Source: CAD feature listing. Evaluate the final solid. Frame: model axes, mm. A direction names the side the tool comes from. Round coordinates to 2 decimals unless told otherwise and drop trailing zeros. Order: outer loops, then holes, each group sorted by start corner. A loop starts at its lowest first (then second) coordinate and runs counter-clockwise, first axis right, second up. Notation, with made-up numbers: M 38.25,77 L 83.25,77 A9 cw 83.25,88 Z; hole C -17,-25 d10. An arc over 180 degrees is marked long. Answer as CSV lines item,"result". Start each with the question number.
Item 1: Section query A-A on x = -25. State how many separate pieces and enclosed holes the cut face has, plus the area to 3 significant figures.
Item 2: Section query B-B on x = -14.5. Return the cut outline in (y, z), plus the area to 3 significant figures.
Item 3: First-contact query: P1, Ø8, axis at x = -17, z = 9, coming from the +Y side; P2, Ø0.8, axis at x = 37, y = -19.5, coming from the +Z side; P3, Ø2.5, axis at x = 25, y = 29.5, coming from the +Z side; P4, Ø13, axis at x = 8.5, z = 8.5, coming from the -Y side. Flat tips, straight axial feed; report the tip coordinate or a pass-through.
Item 4: Pull-direction query (X, two-part tool) for faces 6 (the face through (36.86, -0.9, 18.11)), 7 (the face through (-34.577, 23.748, -1.787)), 8 (the face through (44.748, 11.112, -1.787)); classes: +X half, -X half, draft (parallel to the pull), parting line (faces both ways), or undercut.
Item 5: Section query C-C on x = -2. Return the cut outline in (y, z), plus the area to 3 significant figures.
Item 6: Line query: line 1 (Y direction, x = -33.5, z = 18.25); line 2 (Y direction, x = 25, z = -1.5); line 3 (X direction, y = 3.5, z = 24.75). Output: solid intervals per line, ascending. Write a range as [from, to].
Item 7: Set-up query: faces 1 (the face through (40.96, 18.61, 11.34)), 2 (the face through (43.93, 22.85, 13.18)), 3 (the face through (-24, 27, 0)), 4 (the face through (-26.11, 28.49, -1.76)), 5 (the face through (38.5, -21, 10)). Return all of +Z, -Z, +X, -X, +Y, -Y with unobstructed straight access to the full face (end or side cutting, diameter ignored); none if empty.
from build123d import *

# Parameters (mm, degrees)
PAD_DEPTH       = 26
FILLET_R        = 3
THICKNESS_T     = 2.5
SKETCH001_R     = 2.5
SKETCH001_R_2   = 1
PAD001_DEPTH    = 4
SKETCH007_W     = 19
SKETCH007_H     = 8
POCKET_DEPTH    = 5
PAD008_DEPTH    = 10
SKETCH013_W     = 22
SKETCH013_H     = 10
POCKET002_DEPTH = 5
SKETCH014_W     = 24
SKETCH014_H     = 10
POCKET003_DEPTH = 5
FILLET001_R     = 2
FILLET002_R     = 2
FILLET003_R     = 2
SKETCH015_W     = 5
SKETCH015_H     = 5
SKETCH015_R     = 1
PAD011_DEPTH    = 24
SKETCH016_R     = 1.5
PAD012_DEPTH    = 2.5
CHAMFER_SIZE    = 1
CHAMFER001_SIZE = 1
CHAMFER002_SIZE = 1


with BuildPart() as part:
    # Sketch → Pad (new body)
    with BuildSketch(Plane.XY):
        Polygon((-43, 22), (-43, 0), (-36, 0), (-36, -41), (36, -41), (36, 0), (43, 0), (43, 22), align=None)
    extrude(amount=PAD_DEPTH)

    # Fillet
    fillet_edges = [part.edges().sort_by_distance(p)[0] for p in [
        (-36, -41, 13),
        (36, -41, 13),
        (43, 0, 13),
        (-43, 0, 13),
        (-43, 22, 13),
        (43, 22, 13),
        (36, 0, 13),
        (-36, 0, 13),
    ]]
    fillet(fillet_edges, radius=FILLET_R)

    # Thickness
    thickness_openings = [part.faces().sort_by_distance(p)[0] for p in [
        (0, -8.19552, 26),
    ]]
    offset(amount=THICKNESS_T, openings=thickness_openings)

    # Sketch001 (on Face2 of Thickness) → Pad001 (join)
    with BuildSketch(Plane.XY):
        with Locations((-32.7, -6.5)):
            Circle(SKETCH001_R)
        with Locations((-32.7, -6.5)):
            Circle(SKETCH001_R_2, mode=Mode.SUBTRACT)
        with Locations((-32.7, -32.7)):
            Circle(SKETCH001_R)
        with Locations((-32.7, -32.7)):
            Circle(SKETCH001_R_2, mode=Mode.SUBTRACT)
        with Locations((32.7, -32.7)):
            Circle(SKETCH001_R)
        with Locations((32.7, -32.7)):
            Circle(SKETCH001_R_2, mode=Mode.SUBTRACT)
        with Locations((32.7, -6.5)):
            Circle(SKETCH001_R)
        with Locations((32.7, -6.5)):
            Circle(SKETCH001_R_2, mode=Mode.SUBTRACT)
    extrude(amount=PAD001_DEPTH)

    # Sketch007 (on Face24 of Pad001) → Pocket (cut)
    with BuildSketch(Plane.YZ.offset(38.5)):
        with Locations((-20.85, 22)):
            Rectangle(SKETCH007_W, SKETCH007_H)
    extrude(amount=-POCKET_DEPTH, mode=Mode.SUBTRACT)

    # Sketch009 (on Face2 of Pocket) → Pad008 (join)
    with BuildSketch(Plane.XY):
        Polygon((43, 5), (37.6, 5), (37.6, 1), (30.6, 1), (30.6, -3), (37.6, -3), (43, 0), align=None)
        Polygon((-43, 5), (-37.6, 5), (-37.6, 1), (-30.6, 1), (-30.6, -3), (-37.6, -3), (-43, 0), align=None)
    extrude(amount=PAD008_DEPTH)

    # Sketch013 → Pocket002 (cut)
    with BuildSketch(Plane.XZ.offset(43.5)):
        with Locations((-19, 14.5)):
            Rectangle(SKETCH013_W, SKETCH013_H)
    extrude(amount=-POCKET002_DEPTH, mode=Mode.SUBTRACT)

    # Sketch014 (on Face36 of Pocket002) → Pocket003 (cut)
    with BuildSketch(Plane(origin=(-38.5, 0, 0), x_dir=(0, -1, 0), z_dir=(-1, 0, 0))):
        with Locations((15, 8.5)):
            Rectangle(SKETCH014_W, SKETCH014_H)
    extrude(amount=-POCKET003_DEPTH, mode=Mode.SUBTRACT)

    # Fillet001
    fillet001_edges = [part.edges().sort_by_distance(p)[0] for p in [
        (-37.25, -3, 13.5),
        (-37.25, -3, 3.5),
        (-37.25, -27, 13.5),
        (-37.25, -27, 3.5),
    ]]
    fillet(fillet001_edges, radius=FILLET001_R)

    # Fillet002
    fillet002_edges = [part.edges().sort_by_distance(p)[0] for p in [
        (-30, -42.25, 9.5),
        (-30, -42.25, 19.5),
        (-8, -42.25, 19.5),
        (-8, -42.25, 9.5),
    ]]
    fillet(fillet002_edges, radius=FILLET002_R)

    # Fillet003
    fillet003_edges = [part.edges().sort_by_distance(p)[0] for p in [
        (37.25, -30.35, 18),
        (37.25, -11.35, 18),
    ]]
    fillet(fillet003_edges, radius=FILLET003_R)

    # Sketch015 (on Face10 of Fillet003) → Pad011 (join)
    with BuildSketch(Plane.XY):
        with Locations((-40.5, 19.5)):
            Rectangle(SKETCH015_W, SKETCH015_H)
        with Locations((-40.5, 19.5)):
            Circle(SKETCH015_R, mode=Mode.SUBTRACT)
        with Locations((40.5, 19.5)):
            Rectangle(SKETCH015_W, SKETCH015_H)
        with Locations((40.5, 19.5)):
            Circle(SKETCH015_R, mode=Mode.SUBTRACT)
        with Locations((33.5, -38.5)):
            Rectangle(SKETCH015_W, SKETCH015_H)
        with Locations((33.5, -38.5)):
            Circle(SKETCH015_R, mode=Mode.SUBTRACT)
        with Locations((-33.5, -38.5)):
            Rectangle(SKETCH015_W, SKETCH015_H)
        with Locations((-33.5, -38.5)):
            Circle(SKETCH015_R, mode=Mode.SUBTRACT)
    extrude(amount=PAD011_DEPTH)

    # Sketch016 (on Face110 of Pad011) → Pad012 (join)
    with BuildSketch(Plane(origin=(0, 0, -2.5), x_dir=(1, 0, 0), z_dir=(0, 0, -1))):
        with BuildLine():
            ThreePointArc((-20, 48.5), (-25, 53.5), (-30, 48.5))
            Line((-30, 48.5), (-30, 38.5))
            ThreePointArc((-30, 38.5), (-25, 33.5), (-20, 38.5))
            Line((-20, 48.5), (-20, 38.5))
        make_face()
        with Locations((-25, 48.5)):
            Circle(SKETCH016_R, mode=Mode.SUBTRACT)
        with BuildLine():
            ThreePointArc((30, 48.5), (25, 53.5), (20, 48.5))
            Line((20, 48.5), (20, 38.5))
            ThreePointArc((20, 38.5), (25, 33.5), (30, 38.5))
            Line((30, 48.5), (30, 38.5))
        make_face()
        with Locations((25, 48.5)):
            Circle(SKETCH016_R, mode=Mode.SUBTRACT)
        with BuildLine():
            ThreePointArc((-20, -19.5), (-25, -14.5), (-30, -19.5))
            Line((-30, -19.5), (-30, -29.5))
            ThreePointArc((-30, -29.5), (-25, -34.5), (-20, -29.5))
            Line((-20, -19.5), (-20, -29.5))
        make_face()
        with Locations((-25, -29.5)):
            Circle(SKETCH016_R, mode=Mode.SUBTRACT)
        with BuildLine():
            ThreePointArc((30, -19.5), (25, -14.5), (20, -19.5))
            Line((20, -19.5), (20, -29.5))
            ThreePointArc((20, -29.5), (25, -34.5), (30, -29.5))
            Line((30, -19.5), (30, -29.5))
        make_face()
        with Locations((25, -29.5)):
            Circle(SKETCH016_R, mode=Mode.SUBTRACT)
    extrude(amount=-PAD012_DEPTH)

    # Chamfer
    chamfer_edges = [part.edges().sort_by_distance(p)[0] for p in [
        (-20, -46, 0),
        (20, -46, 0),
        (-30, 27, 0),
        (20, 27, 0),
        (23.5, 29.5, 0),
        (-26.5, 29.5, 0),
        (-26.5, -48.5, 0),
        (23.5, -48.5, 0),
    ]]
    chamfer(chamfer_edges, length=CHAMFER_SIZE)

    # Chamfer001
    chamfer001_edges = [part.edges().sort_by_distance(p)[0] for p in [
        (-41.5, 19.5, 24),
        (39.5, 19.5, 24),
        (32.5, -38.5, 24),
        (-34.5, -38.5, 24),
    ]]
    chamfer(chamfer001_edges, length=CHAMFER001_SIZE)

    # Chamfer002
    chamfer002_edges = [part.edges().sort_by_distance(p)[0] for p in [
        (-37.6, 3, 10),
        (-34.1, 1, 10),
        (34.1, 1, 10),
        (37.6, 3, 10),
    ]]
    chamfer(chamfer002_edges, length=CHAMFER002_SIZE)


solid = part.part
Results:
1,separate pieces,"4"
1,enclosed holes,"0"
1,area,"307 mm^2"
2,outline,"M -43.5,0 A2.5 ccw -41,-2.5 L 22,-2.5 A2.5 ccw 24.5,0 L 24.5,26 L 22,26 L 22,0 L -41,0 L -41,9.5 L -43.5,9.5 Z; M -43.5,19.5 L -41,19.5 L -41,26 L -43.5,26 Z"
2,area,"272 mm^2"
3,P1,"y = 24.5"
3,P2,"z = 18"
3,P3,"through"
3,P4,"y = -43.5"
4,face 6,"undercut"
4,face 7,"draft"
4,face 8,"+X half"
5,outline,"M -43.5,0 A2.5 ccw -41,-2.5 L 22,-2.5 A2.5 ccw 24.5,0 L 24.5,26 L 22,26 L 22,0 L -41,0 L -41,26 L -43.5,26 Z"
5,area,"297 mm^2"
6,line 1,"[-43.48, -39.5], [-37.5, -36], [22, 24.5]"
6,line 2,"[-53.5, -50], [-47, 28], [31, 34.5]"
6,line 3,"[-45.5, -43], [43, 45.5]"
7,face 1,"+Z"
7,face 2,"+Z, -Z, +X, +Y"
7,face 3,"+Z, +X, -X, +Y"
7,face 4,"+Z, -Z"
7,face 5,"+Z, -Z, +X, -Y"
